The figure shows three views and two pictorial views of one solid part (mm, origin at its lowest corner). Answer the questions. Coordinates: 2 decimals unless noted, no trailing zeros. Write each loop counter-clockwise with the first axis right and the second up, starting at its lowest first coordinate (ties: lowest second). Pieces come first, ordered by that corner, then holes. Notation, with made-up numbers: M -24,55.25 L 11,55.25 A9 cw 11,60.25 Z; hole C -29,24.25 d10. An arc over 180 degrees is marked long. Write item = value, one per line.
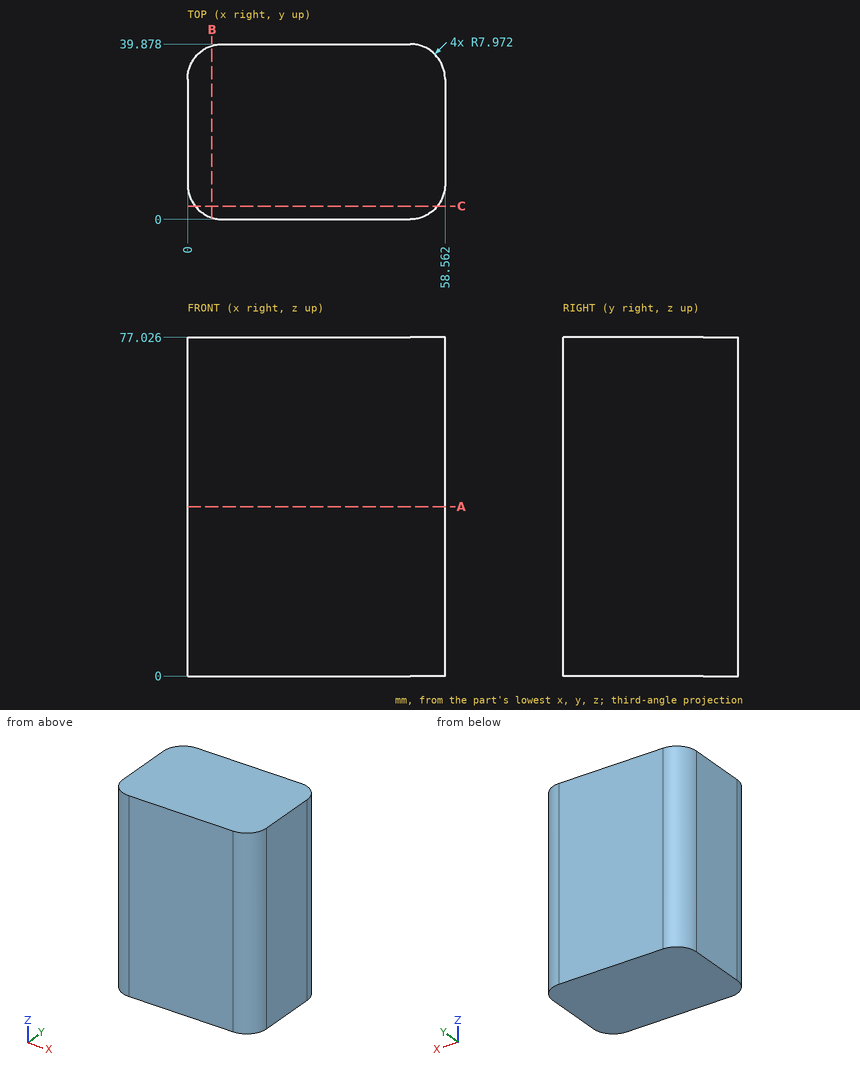
Item 1: Find section C-C (y = 3). Determine the outline of the cut face in (x, z), and give its area (3 significant figures).
Worked answers:
outline = M 1.74,0 L 56.82,0 L 56.82,77.03 L 1.74,77.03 Z
area = 4,240 mm²
Item 2: Consider line 1 along X through (y, z) = (32, 33.5); line 2 along X through (y, z) = (36, 47.5); line 3 along Y through (x, z) = (53, 21.5) (1 decimal). Determine where each line is inside the solid, lowest interval first. Write a range as from..to.
Worked answers:
line_1 = 0..58.56
line_2 = 1.13..57.43
line_3 = 0.4..39.5
Item 3: Find section B-B (x = 5.5). Determine the outline of the cut face in (y, z) (1 decimal).
Worked answers:
outline = M 0.4,0 L 39.5,0 L 39.5,77 L 0.4,77 Z
Item 4: Find section A-A (z = 38.5). Determine the outline of the cut face in (x, y), and give its area (3 significant figures).
Worked answers:
outline = M 0,7.97 A7.97 ccw 7.97,0 L 50.59,0 A7.97 ccw 58.56,7.97 L 58.56,31.91 A7.97 ccw 50.59,39.88 L 7.97,39.88 A7.97 ccw 0,31.91 Z
area = 2,280 mm²
